Source: CAD feature listing. Evaluate the final solid. Frame: model axes, mm. Face numbers are marked on the shaded views. A direction names the side the tool comes from. Give positions to 0.01 mm unless a question says otherwise; leave off trailing zeros. Loops run counter-clockwise (first coordinate to the right, second up) from the corner with the lowest first, then second, coordinate; pieces in that order, holes last. Notation, with made-up numbers: M 28,12 L 70,12 A24 cw 70,22 Z; hole C -3,38 d11. An arc over 180 degrees is marked long. Put each result on its own line as item: value.
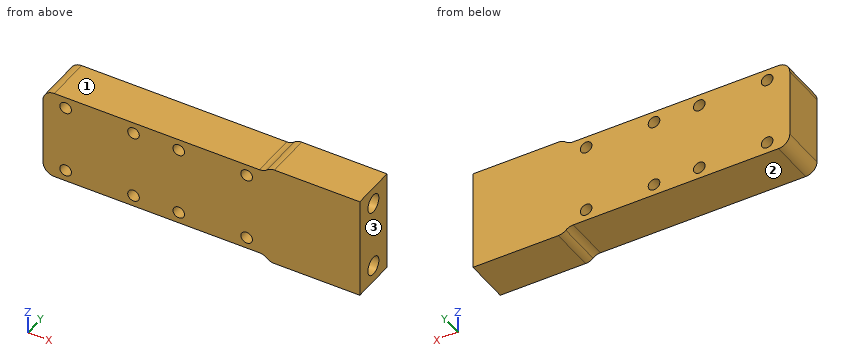
Autodesk Inventor part; units mm, degrees
ref_plane "YZ Plane" through (0, 0, 0) normal (1, 0, 0) x (0, 1, 0)
ref_plane "XZ Plane" through (0, 0, 0) normal (0, 1, 0) x (-1, 0, 0)
ref_plane "XY Plane" through (0, 0, 0) normal (0, 0, 1) x (1, 0, 0)
sketch "Sketch1" plane through (0, 0, 0) normal (0, 1, 0) x (-1, 0, 0)
  line L0 (0, 0) -> (63.5, 0)
  line L1 (63.5, 0) -> (63.5, -25.4)
  line L2 (63.5, -25.4) -> (0, -25.4)
  line L3 (0, -25.4) -> (0, 0) construction
  line L4 (0, 1.5875) -> (-25.4, 1.5875)
  line L5 (-25.4, 1.5875) -> (-25.4, -26.9875)
  line L6 (-25.4, -26.9875) -> (0, -26.9875)
  line L7 (0, -26.9875) -> (0, 1.5875)
  circle A0 centre (6.35, -3.175) radius 1.6256
  circle A1 centre (25.4, -3.175) radius 1.6256
  circle A2 centre (6.35, -22.225) radius 1.6256
  circle A3 centre (25.4, -22.225) radius 1.6256
  circle A4 centre (57.15, -3.175) radius 1.6256
  circle A5 centre (57.15, -22.225) radius 1.6256
  circle A6 centre (38.1, -3.175) radius 1.6256
  circle A7 centre (38.1, -22.225) radius 1.6256
  point P0 (0, -12.7)
  point P1 (0, -12.7)
  point P2 (-12.7, 1.5875)
  point P3 (-12.7, -26.9875)
  point P4 (0, -25.4)
  dimension "d0" = 25.4
  dimension "d11" = 63.5
  dimension "d12" = 25.4
  dimension "d20" = 3.2512
  dimension "d23" = 19.05
  dimension "d26" = 19.05
  dimension "d29" = 3.2512
  dimension "d32" = 19.05
  dimension "d35" = 19.05
  dimension "d38" = 12.7
  dimension "d39" = 6.35
  dimension "d40" = 3.175
  dimension "d41" = 28.575
extrude "Extrusion1" add sketch "Sketch1" along normal blind 12.7
fillet "Fillet1" radius 3.175 6 edges at (-63.5, 6.35, -25.4) (-63.5, 6.35, 0) (0, 6.35, -25.4) (0, 6.35, -26.9875) (0, 6.35, 0) (0, 6.35, 1.5875)
sketch "Sketch2" plane through (25.4, 0, 1.5875) normal (1, 0, 0) x (0, 0, -1)
  line L0 (0, 12.7) -> (28.575, 12.7)
  line L1 (28.575, 12.7) -> (28.575, 0)
  line L2 (28.575, 0) -> (0, 0)
  line L3 (0, 0) -> (0, 12.7)
  line L4 (0, 12.7) -> (28.575, 0) construction
  line L5 (28.575, 12.7) -> (0, 0) construction
  line L6 (0, 12.7) -> (28.575, 12.7)
  line L7 (0, 0) -> (0, 12.7)
  circle A0 centre (23.8125, 6.35) radius 2.5527
  circle A1 centre (4.7625, 6.35) radius 2.5527
  point P0 (1.5875, 0)
  point P1 (14.2875, 6.35)
  dimension "d45" = 5.1054
  dimension "d46" = 9.525
  dimension "d47" = 9.525
extrude "Extrusion2" cut sketch "Sketch2" against normal blind 25.4 contours A0 | A1
thread "Thread1"
thread "Thread2"
properties part number "DVBS_009_RemoteLookingBracket" material "Polyethylene, High Density"
1. Section query C-C (x = -38.1). Output: boundary loops of the cut face in (y, z).
Found:
outline: M 0,-25.4 L 12.7,-25.4 L 12.7,-23.85 L 0,-23.85 Z; M 0,-20.6 L 12.7,-20.6 L 12.7,-4.8 L 0,-4.8 Z; M 0,-1.55 L 12.7,-1.55 L 12.7,0 L 0,0 Z
2. Contact query for flat-ended pins moving along their axis: P1, Ø6.5, axis at x = -35, y = 8, coming from the +Z side; P2, Ø4, axis at x = -37.5, y = 4, coming from the -Z side; P3, Ø1.5, axis at y = 5.5, z = -4, coming from the +X side. Output: stop coordinate, or through.
Found:
P1: z = 0
P2: z = -25.4
P3: x = 0
3. Section query A-A (y = 10.5). State how many separate pieces and enclosed holes the cut face has, plus the area to 3 significant figures.
Found:
separate pieces: 1
enclosed holes: 8
area: 2,270 mm^2
4. Material intervals for line 1 (Z direction, x = -25.4, y = 4.5); line 2 (X direction, y = 3, z = -22.25); line 3 (Z direction, x = -6.5, y = 12), sorted ascending. Write a range as from..to.
Found:
line 1: -25.4..-23.85, -20.6..-4.8, -1.55..0
line 2: -63.5..-58.78, -55.52..-39.73, -36.47..-27.03, -23.77..-7.98, -4.72..25.4
line 3: -25.4..-23.84, -20.61..-4.79, -1.56..0
5. Access query for the marked faces 1, 2 and 3. Directions: +Z, -Z, +X, -X, +Y, -Y. A direction counts if a zero-diameter tool reaches every point of the face in a straight line with its end or side. Return the directions, or none.
Found:
face 1: +Z, -X, +Y, -Y
face 2: -Z, -X, +Y, -Y
face 3: +Z, -Z, +X, +Y, -Y
